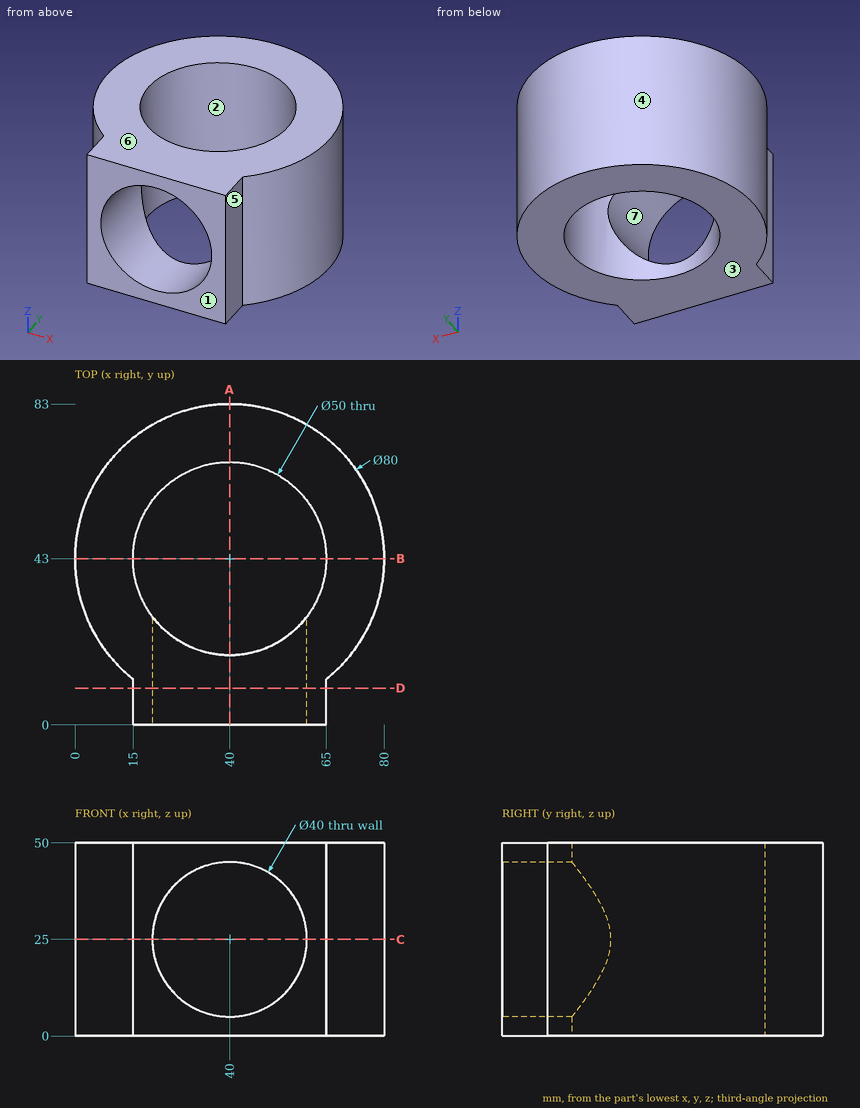
Geometry: see drawing. Coordinates: mm, zero at the bounding-box minimum. A direction names the side the tool comes from. Round coordinates to 2 decimals unless told otherwise and drop trailing zeros. Write each loop counter-clockwise with the first axis right and the second up, starting at its lowest first coordinate (ties: lowest second). Pieces come first, ordered by that corner, then holes. Notation, with made-up numbers: M -40,80.25 L -6,80.25 A31 cw -6,112.25 Z; hole C 81.5,16.5 d3. An arc over 180 degrees is marked long. Answer in a Markdown table with one row per item. Add a question column.
(1) Cut plane A-A, the plane x = 40. Return the cut outline in (y, z).
(2) Draft query along Y for the marked faces 1, 2, 3 and 4. Return one class per face: pulls with the +Y half, pulls with the -Y half, needs draft (parallel to the pull), parting line crosses it, or undercut.
(3) Cut plane C-C, the plane z = 25. Return the cut outline in (x, y) (3 decimals).
(4) Contact query for flat-ended pins moving along their axis: pin 1 (4 mm diameter, centred on x = 43, z = 30, fed in from -Y); pin 2 (3.5 mm diameter, centred on y = 6, z = 19, fed in from +X); pin 3 (13 mm diameter, centred on y = 7, z = 21, fed in from -X). Output: stop coordinate, or through.
(5) Cut plane B-B, the plane y = 43. Return the cut outline in (x, z).
(6) Ray query, L1, parallel to Z at x = 40, y = 12.75; L2, parallel to Y at x = 40, z = 32; L3, parallel to X at y = 30, z = 37. Return the intervals inside material, ascending.
(7) Cut plane D-D, the plane y = 9.5. Return the cut outline in (x, z).
(8) Reachability of the marked faces 5, 6 and 7 from +Z, -Z, +X, -X, +Y, -Y: full face, straight path, thin tool, end or side. Return the list, or none.
Established:
| question | item | result |
|---|---|---|
| 1 | outline | M 0,0 L 18,0 L 18,5 L 0,5 Z; M 0,45 L 18,45 L 18,50 L 0,50 Z; M 68,0 L 83,0 L 83,50 L 68,50 Z |
| 2 | face 1 | pulls with the -Y half |
| 2 | face 2 | undercut |
| 2 | face 3 | needs draft |
| 2 | face 4 | parting line crosses it |
| 3 | outline | M 15,0 L 20,0 L 20,28 A25 cw long 60,28 L 60,0 L 65,0 L 65,11.775 A40 ccw long 15,11.775 Z |
| 4 | pin 1 | y = 67.49 |
| 4 | pin 2 | x = 65 |
| 4 | pin 3 | x = 12.99 |
| 5 | outline | M 0,0 L 15,0 L 15,50 L 0,50 Z; M 65,0 L 80,0 L 80,50 L 65,50 Z |
| 6 | L1 | 0 to 5, 45 to 50 |
| 6 | L2 | 68 to 83 |
| 6 | L3 | 2.17 to 18.65, 61.35 to 77.83 |
| 7 | outline | M 15,0 L 65,0 L 65,50 L 15,50 Z; hole C 40,25 d40 |
| 8 | face 5 | +Z, -Z, +X, -Y |
| 8 | face 6 | +Z, +X, -X, +Y, -Y |
| 8 | face 7 | -Y |
